Answer from the drawing. Dimensions are ordinates in mm from the lowest x, y and z of the part. Round coordinates to 2 decimals unless told otherwise and drop trailing zeros. Loops run counter-clockwise (first coordinate to the right, second up) from the corner with the lowest first, then second, coordinate; pieces in that order, holes last.
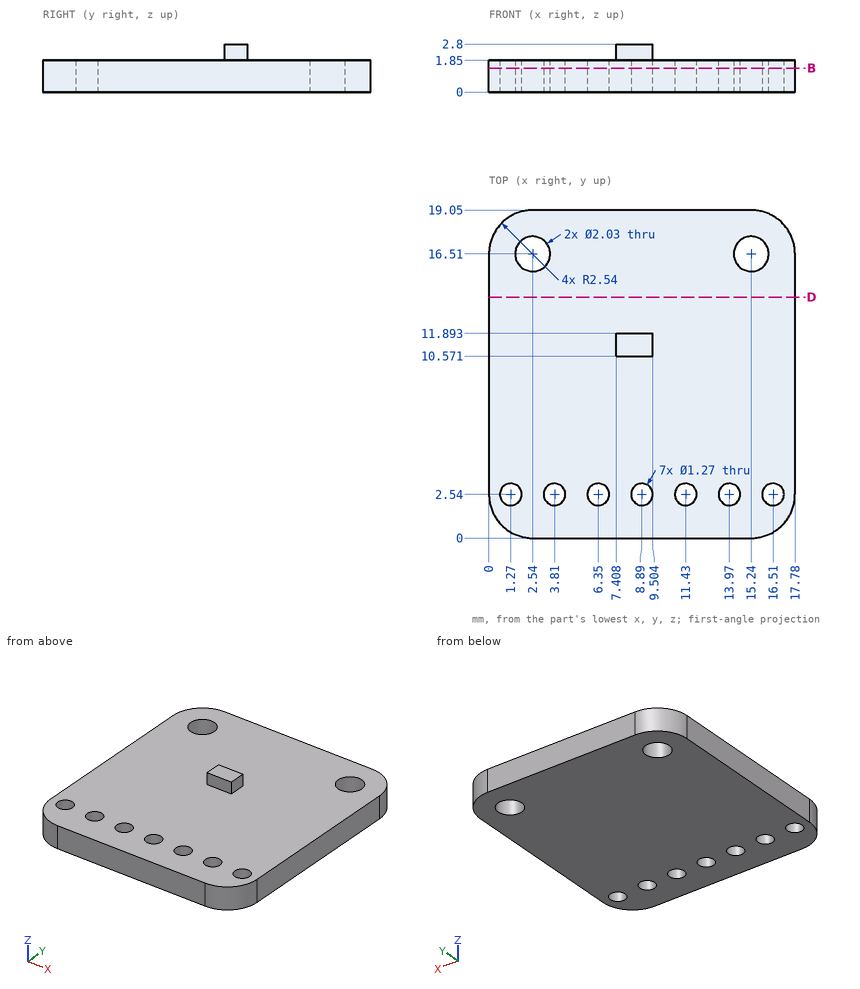
1. Find section B-B (z = 1.4). Give the number of separate pieces and of enclosed holes in the cut face, then the cut area to 3 significant figures.
Answer key:
separate pieces: 1
enclosed holes: 9
area: 318 mm2
2. Consider probe 1 along Z at (x, y) = (13.5, 13); probe 2 along X at (y, z) = (11, 2.35); probe 3 along Y at (x, z) = (16.51, 1.2) (1 decimal). Determine where each line is inside the solid, lowest interval first.
Answer key:
probe 1: z = 0 to 1.85
probe 2: x = 7.41 to 9.5
probe 3: y = 0.3 to 1.9, 3.2 to 18.7
3. Given pin 1 (0.8 mm diameter, centred on x = 13.97, y = 2.54, fed in from -Z); pin 2 (2.5 mm diameter, centred on x = 15.24, y = 16.51, fed in from +Z); pin 3 (0.5 mm diameter, centred on y = 11.5, z = 2.5, fed in from +X), each flat-ended and moving along its own axis, determine where each tip first touches the part or whether it passes through.
Answer key:
pin 1: passes through
pin 2: stops at z = 1.85
pin 3: stops at x = 9.5
4. Find section D-D (y = 14). Write down the section's boundary in (x, z).
Answer key:
outline: (0, 0) - (17.78, 0) - (17.78, 1.85) - (0, 1.85) - close
